Can you work these out from the model? Positions are in its coordinate system, mm. A direction names the side the tool comes from. Coordinates: 2 decimals unless noted, no trailing zeros. Order: outer loops, then holes, each group sorted by start corner. A loop starts at its lowest first (then second) coordinate and runs counter-clockwise, first axis right, second up. Notation, with made-up numbers: (19.25, 51.5) -> (51.25, 51.5) arc R32 ccw to (51.25, 78.5) -> close; hole circle Ø8 at (61.5, -19.5). An arc over 180 degrees is marked (long way). Use a Markdown table: item, result. Add a question column.
1. Suppose I cut it at D-D, the plane x = -21. List the corners of the cut face in (y, z) for me (3 decimals), then the cut area to 3 significant figures.
2. Suppose I cut it at C-C, the plane y = -9.5. List the corners of the cut face in (x, z) for me.
3. We'd pull the mould along Y, two halves only. Please class faces 1 (the flat face through (-2, 3.175, 8)), 2 (the flat face through (2, -3.175, 8)), 3 (the flat face through (0, 1.651, 9)), 4 (the flat face through (-22.225, -2, 34)): pulls with the +Y half, pulls with the -Y half, needs draft (parallel to the pull), parting line crosses it, or undercut.
4. For faces 5 (the flat face through (0, -15, 5)), 6 (the flat face through (22.225, 2, 34)), 7 (the flat face through (0, 16, 5)), 8 (the flat face through (0, -1.651, 9)), which set-ups out of +Z, -Z, +X, -X, +Y, -Y let a thin tool reach every point of the face, with its end or its side?
5. Suppose I cut it at A-A, the plane x = 0. List the corners of the cut face in (y, z) for me (3 decimals).
6. If I drill on line 1 along X through (y, z) = (1, 24); line 2 along Y through (x, z) = (0, 1.75); line 3 along Z through (x, y) = (-9, 11), over which ranges is the centre line in solid material (lowest first)? Write a range as from..to.
7. Suppose I cut it at B-B, the plane z = 20.5. List the corners of the cut face in (x, y) for me (3 decimals).
8. For pin 1 Ø1.5 at (y, z) = (2, 13) entering from -X; pin 2 Ø0.8 at (x, y) = (-2.5, -2.5) entering from -Z; pin 3 Ø0.5 at (y, z) = (2.5, 26) entering from +X; pin 4 Ø4 at (y, z) = (-5.5, 51) entering from +X, each with a flat end and sliding along its axis, tell me the tip position at first contact or that it passes through.
```python
from build123d import *

# Parameters (mm, degrees)
F0_R     = 27.94
F1_DEPTH = 5
F3_DEPTH = 52.054
F4_W     = 50.8
F4_H     = 3.302
F5_DEPTH = 50.8
F6_W     = 44.45
F6_H     = 6.35
F7_DEPTH = 47.625
F8_R     = 11
F9_DEPTH = 7


with BuildPart() as f1:
    # F0 (on Top) → F1 (new body)
    with BuildSketch(Plane.XY):
        Circle(F0_R)
    extrude(amount=F1_DEPTH)

    # F2 (on face) → F3 (join)
    with BuildSketch(Plane.XY.offset(5)):
        with BuildLine():
            ThreePointArc((27.94, 0), (27.8947173307, 1.5900770556), (27.7590161029, 3.175))
            Line((27.7590161029, 3.175), (-27.7590161029, 3.175))
            ThreePointArc((-27.7590161029, 3.175), (-27.8947173307, 1.5900770556), (-27.94, 0))
            ThreePointArc((-27.94, 0), (-27.8947173307, -1.5900770556), (-27.7590161029, -3.175))
            Line((-27.7590161029, -3.175), (27.7590161029, -3.175))
            ThreePointArc((27.7590161029, -3.175), (27.8947173307, -1.5900770556), (27.94, 0))
        make_face()
    extrude(amount=F3_DEPTH)

    # F4 (on face) → F5 (cut)
    with BuildSketch(Plane.XY.offset(57.054)):
        Rectangle(F4_W, F4_H)
    extrude(amount=-F5_DEPTH, mode=Mode.SUBTRACT)

    # F6 (on face) → F7 (cut)
    with BuildSketch(Plane.XY.offset(57.054)):
        Rectangle(F6_W, F6_H)
    extrude(amount=-F7_DEPTH, mode=Mode.SUBTRACT)

    # F8 (on face) → F9 (cut)
    with BuildSketch(Plane(origin=(0, 0, 0), x_dir=(1, 0, 0), z_dir=(0, 0, -1))):
        Circle(F8_R)
    extrude(amount=-F9_DEPTH, mode=Mode.SUBTRACT)


solid = f1.part
```
Worked out:
| question | item | result |
|---|---|---|
| 1 | outline | (-18.429, 0) -> (18.429, 0) -> (18.429, 5) -> (3.175, 5) -> (3.175, 9.429) -> (1.651, 9.429) -> (1.651, 6.254) -> (-1.651, 6.254) -> (-1.651, 9.429) -> (-3.175, 9.429) -> (-3.175, 5) -> (-18.429, 5) -> close |
| 1 | area | 202 mm² |
| 2 | outline | (-26.28, 0) -> (-5.55, 0) -> (-5.55, 5) -> (-26.28, 5) -> close; (5.55, 0) -> (26.28, 0) -> (26.28, 5) -> (5.55, 5) -> close |
| 3 | face 1 | pulls with the +Y half |
| 3 | face 2 | pulls with the -Y half |
| 3 | face 3 | undercut |
| 3 | face 4 | needs draft |
| 4 | face 5 | +Z, +X, -X, -Y |
| 4 | face 6 | +Z, +Y, -Y |
| 4 | face 7 | +Z, +X, -X, +Y |
| 4 | face 8 | +Z |
| 5 | outline | (-27.94, 0) -> (-11, 0) -> (-11, 5) -> (-27.94, 5) -> close; (-3.175, 7) -> (-1.651, 7) -> (-1.651, 9.429) -> (-3.175, 9.429) -> close; (1.651, 7) -> (3.175, 7) -> (3.175, 9.429) -> (1.651, 9.429) -> close; (11, 0) -> (27.94, 0) -> (27.94, 5) -> (11, 5) -> close |
| 6 | line 1 | x = -27.92..-25.4, 25.4..27.92 |
| 6 | line 2 | y = -27.94..-11, 11..27.94 |
| 6 | line 3 | z = 0..5 |
| 7 | outline | (-27.759, -3.175) -> (-22.225, -3.175) -> (-22.225, -1.651) -> (-25.4, -1.651) -> (-25.4, 1.651) -> (-22.225, 1.651) -> (-22.225, 3.175) -> (-27.759, 3.175) arc R27.94 ccw to start; (22.225, -3.175) -> (27.759, -3.175) arc R27.94 ccw to (27.759, 3.175) -> (22.225, 3.175) -> (22.225, 1.651) -> (25.4, 1.651) -> (25.4, -1.651) -> (22.225, -1.651) -> close |
| 8 | pin 1 | stops at x = -27.91 |
| 8 | pin 2 | stops at z = 7 |
| 8 | pin 3 | stops at x = 27.85 |
| 8 | pin 4 | passes through |
